```python
from build123d import *

# Parameters (mm, degrees)
BOSS_EXTRUDE6_DEPTH = 1
BOSS_EXTRUDE8_DEPTH = 15


with BuildPart() as part:
    # Sketch1 → Boss-Extrude6 (new body)
    with BuildSketch(Plane(origin=(0, 0, 0), x_dir=(1, 0, 0), z_dir=(0, 1, 0))):
        Polygon((231.716666588, -139.412373829), (462.829865412, -139.412373829), (465.38624875, -134.984588004), (349.829542096, 65.165499075), (344.716133219, 65.165499075), (229.159432538, -134.984249178), align=None)
    extrude(amount=BOSS_EXTRUDE6_DEPTH)

    # Sketch1<7> → Boss-Extrude8 (add)
    with BuildSketch(Plane(origin=(0, 0, 0), x_dir=(1, 0, 0), z_dir=(0, 1, 0))):
        Polygon((351.272917769, 67.665499075), (468.273000096, -134.984588004), (464.273241085, -141.912373829), (230.273290915, -141.912373829), (226.272682946, -134.984246139), (343.272757546, 67.665499075), align=None)
        Polygon((231.716666588, -139.412373829), (462.829865412, -139.412373829), (465.38624875, -134.984588004), (349.829542096, 65.165499075), (344.716133219, 65.165499075), (229.159432538, -134.984249178), align=None, mode=Mode.SUBTRACT)
    extrude(amount=BOSS_EXTRUDE8_DEPTH)


solid = part.part
```
Geometry check sheet. Reference: the model listing, model coordinates, mm. A direction names the side the tool comes from. Coordinates: 2 decimals unless noted, no trailing zeros. Loops run counter-clockwise (first coordinate to the right, second up) from the corner with the lowest first, then second, coordinate; pieces in that order, holes last. Notation, with made-up numbers: (-36.5, 81.25) -> (19.5, 81.25) arc R19 cw to (19.5, 115.25) -> close; hole circle Ø2 at (48.5, 13.25). An arc over 180 degrees is marked (long way). Put each result on its own line as item: value.
1) Gauge pin test, flat ends, axial feed: pin 1 Ø1.5 at (y, z) = (11.5, 74) entering from +X; pin 2 Ø5 at (y, z) = (9.5, 14) entering from +X; pin 3 Ø5 at (x, z) = (271, 110) entering from -Y; pin 4 Ø1 at (y, z) = (10, 84) entering from +X. Record the tip position at first contact, or that the pin passes through.
Result set:
pin 1: stops at x = 433.5
pin 2: stops at x = 399.87
pin 3: stops at y = 0
pin 4: stops at x = 439.13
2) Thickness scan on line 1 (Z direction, x = 347.5, y = 6); line 2 (X direction, y = 11, z = 133); line 3 (Z direction, x = 306, y = 4.5). Record the ranges inside material, lowest first.
Result set:
line 1: z = -67.67 to -65.17, 139.41 to 141.91
line 2: x = 227.42 to 230.31, 464.24 to 467.13
line 3: z = -3.11 to 1.89, 139.41 to 141.91
3) Cross-section at B-B on z = 72.5. Record the boundary of the cut face in (x, y), plus the area to 3 significant figures.
Result set:
outline: (262.35, 0) -> (432.2, 0) -> (432.2, 15) -> (429.31, 15) -> (429.31, 1) -> (265.23, 1) -> (265.23, 15) -> (262.35, 15) -> close
area: 251 mm^2
4) Tool access check on faces 4 (the flat face through (408.417, 7.902, 36.311)), 5 (the flat face through (349, 7, 141.912)). Record the directions out of +Z, -Z, +X, -X, +Y, -Y that give a thin tool (end or side, any length) a straight path to the whole face; none if there is none.
Result set:
face 4: +Y
face 5: +Z, +X, -X, +Y, -Y
5) Cross-section at A-A on y = 4.25. Record the boundary of the cut face in (x, z), plus the area to 3 significant figures.
Result set:
outline: (226.27, 134.98) -> (343.27, -67.67) -> (351.27, -67.67) -> (468.27, 134.98) -> (464.27, 141.91) -> (230.27, 141.91) -> close; hole (229.16, 134.98) -> (344.72, -65.17) -> (349.83, -65.17) -> (465.39, 134.98) -> (462.83, 139.41) -> (231.72, 139.41) -> close
area: 1,790 mm^2
6) Release check for a two-part mould opening along X. For faces 1 (the flat face through (466.3, 7.4, 138.4)), 2 (the flat face through (346, 1, 58)), 3 (the flat face through (349, 0, 59)) record: released by +X, released by -X, zero draft, split by the parting line, or undercut.
Result set:
face 1: released by +X
face 2: undercut
face 3: zero draft
7) Cross-section at C-C on x = 311.5. Record the boundary of the cut face in (y, z).
Result set:
outline: (0, -12.63) -> (15, -12.63) -> (15, -7.63) -> (1, -7.63) -> (1, 139.41) -> (15, 139.41) -> (15, 141.91) -> (0, 141.91) -> close
